Drawing for the job (mm, zero at the part's lowest x, y, z). A direction names the side the tool comes from. Coordinates: 2 decimals unless noted, no trailing zeros. Write each loop counter-clockwise with the first axis right and the second up, starting at its lowest first coordinate (ties: lowest second). Pieces come first, ordered by that corner, then holes. Notation, with made-up numbers: M -9,29 L 36,29 A19 cw 36,46 Z; hole C 43.5,14.5 d4. An arc over 180 degrees is marked long. Put each result on its own line as item: value. Start each with the question number.
Q1. Cut at B-B (x = 25). Write the cut outline in (y, z).
Q2. Cut at D-D (y = 4). Write the cut outline in (x, z), then the cut area to 3 significant figures.
Q3. Cut at A-A (y = 18.5). Write the cut outline in (x, z), then the cut area to 3 significant figures.
Q4. Drop flat-ended pins along their axis: pin 1 (13 mm diameter, centred on x = 25.17, y = 25, fed in from +Z); pin 2 (10 mm diameter, centred on y = 21.5, z = 8, fed in from -X); pin 3 (4 mm diameter, centred on y = 16, z = 13.5, fed in from +X). Give the stop position or say it passes through.
Q5. Which spindle directions (+Z, -Z, +X, -X, +Y, -Y) get a long thin tool onto all of the face, cutting with end or side? Do the marked faces 1, 2, 3, 4 and 5. Say none if no direction does.
Q6. Pull direction Z, two halves, no side cores. Call the marked faces 6, 7, 8 and 9: pulls with the +Z half, pulls with the -Z half, needs draft (parallel to the pull), parting line crosses it, or undercut.
Q7. Drill centre lines: line 1 along Z through (x, y) = (30.5, 21.5); line 2 along Y through (x, z) = (25.5, 27); line 3 along Y through (x, z) = (33.5, 24.5). Where is each one in solid material? Low to high.
Q8. Cut at C-C (z = 3). Write the cut outline in (x, y).
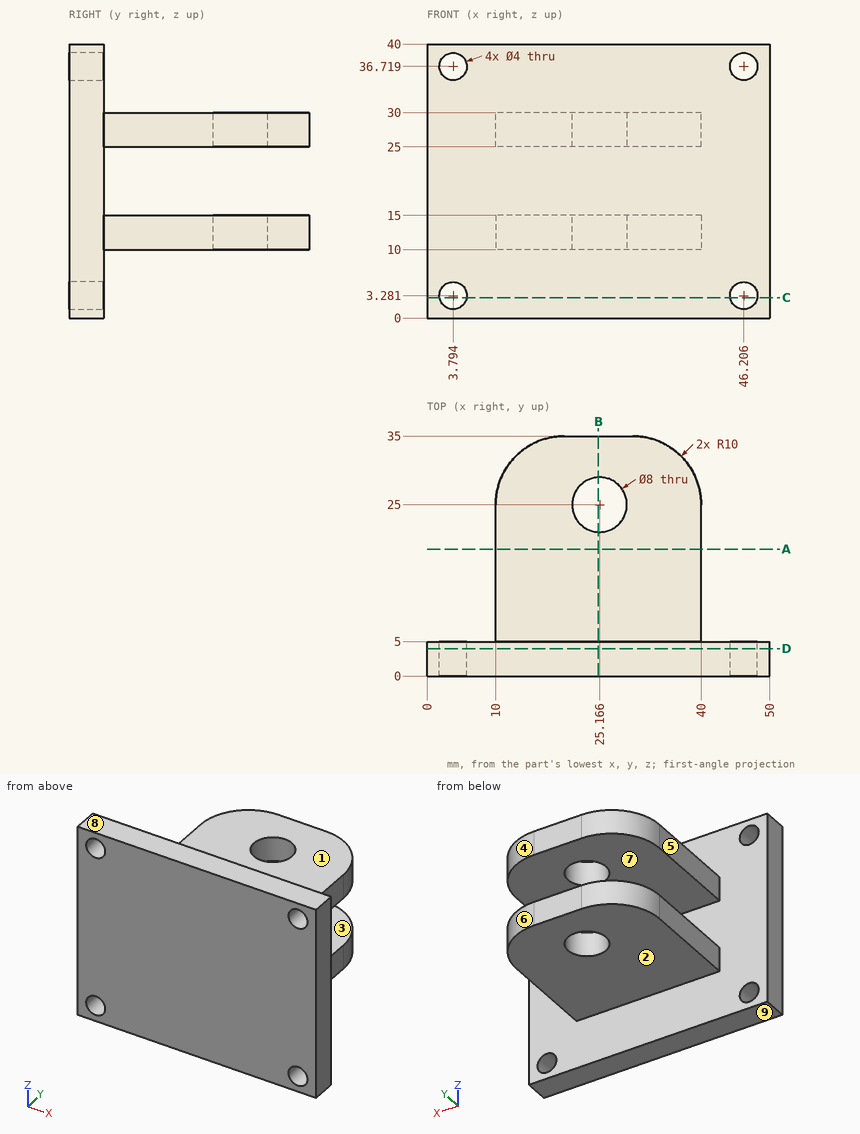
Computed values:
1. outline: M 0,0 L 5,0 L 5,10 L 21,10 L 21,15 L 5,15 L 5,25 L 21,25 L 21,30 L 5,30 L 5,40 L 0,40 Z; M 29,10 L 35,10 L 35,15 L 29,15 Z; M 29,25 L 35,25 L 35,30 L 29,30 Z
2. outline: M 0,0 L 50,0 L 50,40 L 0,40 Z; hole C 3.79,3.28 d4; hole C 3.79,36.72 d4; hole C 46.21,3.28 d4; hole C 46.21,36.72 d4
2. area: 1,950 mm2
3. outline: M 10,10 L 40,10 L 40,15 L 10,15 Z; M 10,25 L 40,25 L 40,30 L 10,30 Z
3. area: 300 mm2
4. pin 1: z = 30
4. pin 2: x = 10
4. pin 3: x = 40
5. face 1: +Z, +X, -X, +Y
5. face 2: -Z, +X, -X, +Y
5. face 3: +X, -X, +Y
5. face 4: +Z, -Z, +X, +Y
5. face 5: +Z, -Z, -X, +Y
6. face 6: needs draft
6. face 7: undercut
6. face 8: pulls with the +Z half
6. face 9: pulls with the -Z half
7. line 1: 10 to 15, 25 to 30
7. line 2: 0 to 21.01, 28.99 to 35
7. line 3: 0 to 5
8. outline: M 0,0 L 1.81,0 L 1.81,5 L 0,5 Z; M 5.77,0 L 44.23,0 L 44.23,5 L 5.77,5 Z; M 48.19,0 L 50,0 L 50,5 L 48.19,5 Z
